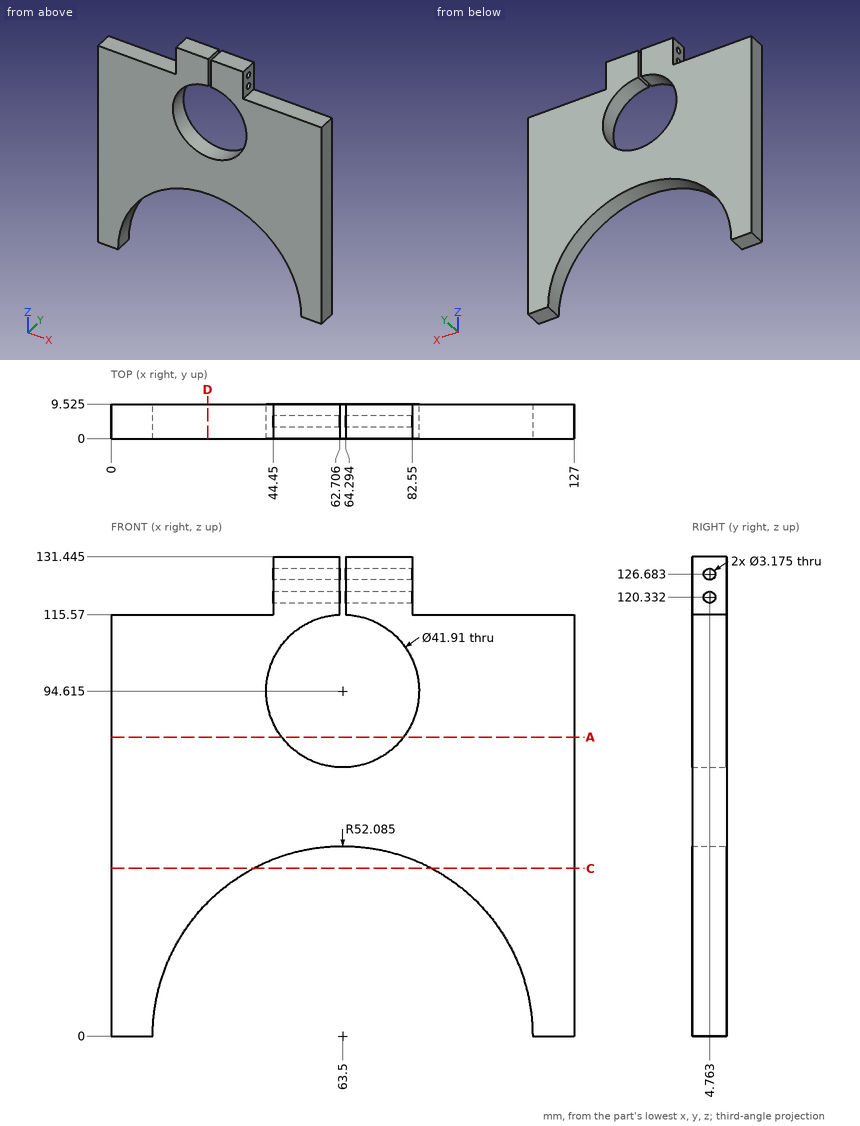
Input: dimensioned drawing with shaded views. Units: mm. Origin: part minimum x, y, z. Round coordinates to 2 decimals unless told otherwise and drop trailing zeros. Order: outer loops, then holes, each group sorted by start corner. A loop starts at its lowest first (then second) coordinate and runs counter-clockwise, first axis right, second up. Notation, with made-up numbers: (24, -25) -> (82, -25) arc R6 ccw to (82, -21) -> close; hole circle Ø4 at (89, 66.5). An arc over 180 degrees is marked (long way). One line per item, written item: value. Start each with the question number.
Q1. Pin query (flat end, axial travel): pin 1 (4 mm diameter, centred on x = 33, y = 5.5, fed in from +Z); pin 2 (1 mm diameter, centred on x = 57.5, y = 7, fed in from -Z); pin 3 (5 mm diameter, centred on y = 4.76, z = 126.68, fed in from -X); pin 4 (12 mm diameter, centred on x = 105.5, z = 24, fed in from -Y). Return the tip coordinate at first contact, or that it passes through.
Q2. Section query A-A (z = 82). Return the cut outline in (x, y) (1 decimal).
Q3. Material intervals for probe 1 along Z at (x, y) = (80, 5.25) (1 decimal); probe 2 along X at (y, z) = (4, 95); probe 3 along X at (y, z) = (1.25, 121.5), sorted ascending.
Q4. Section query C-C (z = 46). Return the cut outline in (x, y) (1 decimal), plus the area to 3 significant figures.
Q5. Section query D-D (x = 26.5). Return the cut outline in (y, z) (1 decimal).
Findings below:
1. pin 1: z = 115.57
1. pin 2: z = 51.68
1. pin 3: x = 44.45
1. pin 4: y = 0
2. outline: (0, 0) -> (46.8, 0) -> (46.8, 9.5) -> (0, 9.5) -> close; (80.2, 0) -> (127, 0) -> (127, 9.5) -> (80.2, 9.5) -> close
3. probe 1: 49.4 to 81.7, 107.5 to 118.8, 121.8 to 125.2, 128.2 to 131.4
3. probe 2: 0 to 42.55, 84.45 to 127
3. probe 3: 44.45 to 62.71, 64.29 to 82.55
4. outline: (0, 0) -> (39.1, 0) -> (39.1, 9.5) -> (0, 9.5) -> close; (87.9, 0) -> (127, 0) -> (127, 9.5) -> (87.9, 9.5) -> close
4. area: 744 mm²
5. outline: (0, 36.7) -> (9.5, 36.7) -> (9.5, 115.6) -> (0, 115.6) -> close
